Here's how the part is built. I have some questions about the finished solid (model axes, mm). Give positions to 0.01 mm unless a question says otherwise; leave off trailing zeros. Loops run counter-clockwise (first coordinate to the right, second up) from the corner with the lowest first, then second, coordinate; pieces in that order, holes last. Notation, with made-up numbers: (2, 73) -> (28, 73) arc R10 cw to (28, 79) -> close; hole circle Ø3 at (2.5, -16.75). An arc over 180 degrees is marked (long way). Answer in a Markdown table with one row per item. Add a question column.
Item 1: If we section it at B-B (z = -5): Write out the boundary of the cut face in (x, y) (3 decimals), then the cut area to 3 significant figures.
Item 2: If I drill on line 1 (Z direction, x = 25, y = -1.8); line 2 (Z direction, x = 23.75, y = -1.7), over which ranges is the centre line in solid material (lowest first)?
Item 3: If we section it at D-D (z = -16): Write out the boundary of the cut face in (x, y) (3 decimals).
Item 4: If we section it at C-C (y = -1.4): Give the number of separate pieces and of enclosed holes in the cut face, then the cut area to 3 significant figures.
Item 5: If we section it at A-A (x = 15): Write out the boundary of the cut face in (y, z) (3 decimals).
Item 6: For P1, Ø3.5, axis at x = 15, z = -15, coming from the -Y side (3 decimals); P2, Ø3, axis at x = 25, z = -35, coming from the +Y side, each with a flat end and sliding along its axis, tell me the tip position at first contact or that it passes through.
Item 7: We'd pull the mould along Z, two halves only. Please class faces 1 (the face through (13.4, -1.57, -24.93)), 2 (the face through (15, -3.175, -20)), 3 (the face through (15, -2, 0)): released by +Z, released by -Z, zero draft, split by the parting line, or undercut.
```python
from build123d import *

# Parameters (mm, degrees)
F0_R     = 1.6
F1_DEPTH = 3.175


# Not quite as in the source:
# - a length typed as a fraction of an inch, garbled in the dataset ("3 / 203.2 mm" for 3/8 in), is restored


with BuildPart() as f1:
    # F0 (on Front) → F1 (new body)
    with BuildSketch(Plane.XZ):
        with BuildLine():
            Line((27.46, 0), (2.54, 0))
            ThreePointArc((2.54, 0), (0.7439487758, -0.7439487758), (0, -2.54))
            Line((0, -2.54), (0, -37.46))
            ThreePointArc((0, -37.46), (0.7439487758, -39.2560512242), (2.54, -40))
            Line((2.54, -40), (27.46, -40))
            ThreePointArc((27.46, -40), (29.2560512242, -39.2560512242), (30, -37.46))
            Line((30, -37.46), (30, -2.54))
            ThreePointArc((30, -2.54), (29.2560512242, -0.7439487758), (27.46, 0))
        make_face()
        with Locations((5, -35)):
            Circle(F0_R, mode=Mode.SUBTRACT)
        with Locations((5, -25)):
            Circle(F0_R, mode=Mode.SUBTRACT)
        with Locations((15, -35)):
            Circle(F0_R, mode=Mode.SUBTRACT)
        with Locations((25, -35)):
            Circle(F0_R, mode=Mode.SUBTRACT)
        with Locations((15, -25)):
            Circle(F0_R, mode=Mode.SUBTRACT)
        with Locations((25, -25)):
            Circle(F0_R, mode=Mode.SUBTRACT)
        with Locations((5, -15)):
            Circle(F0_R, mode=Mode.SUBTRACT)
        with Locations((5, -5)):
            Circle(F0_R, mode=Mode.SUBTRACT)
        with Locations((15, -15)):
            Circle(F0_R, mode=Mode.SUBTRACT)
        with Locations((25, -15)):
            Circle(F0_R, mode=Mode.SUBTRACT)
        with Locations((15, -5)):
            Circle(F0_R, mode=Mode.SUBTRACT)
        with Locations((25, -5)):
            Circle(F0_R, mode=Mode.SUBTRACT)
    extrude(amount=F1_DEPTH)


solid = f1.part
```
Recorded:
| question | item | result |
|---|---|---|
| 1 | outline | (0, -3.175) -> (3.4, -3.175) -> (3.4, 0) -> (0, 0) -> close; (6.6, -3.175) -> (13.4, -3.175) -> (13.4, 0) -> (6.6, 0) -> close; (16.6, -3.175) -> (23.4, -3.175) -> (23.4, 0) -> (16.6, 0) -> close; (26.6, -3.175) -> (30, -3.175) -> (30, 0) -> (26.6, 0) -> close |
| 1 | area | 64.8 mm^2 |
| 2 | line 1 | z = -40 to -36.6, -33.4 to -26.6, -23.4 to -16.6, -13.4 to -6.6, -3.4 to 0 |
| 2 | line 2 | z = -40 to -36, -34 to -26, -24 to -16, -14 to -6, -4 to 0 |
| 3 | outline | (0, -3.175) -> (3.751, -3.175) -> (3.751, 0) -> (0, 0) -> close; (6.249, -3.175) -> (13.751, -3.175) -> (13.751, 0) -> (6.249, 0) -> close; (16.249, -3.175) -> (23.751, -3.175) -> (23.751, 0) -> (16.249, 0) -> close; (26.249, -3.175) -> (30, -3.175) -> (30, 0) -> (26.249, 0) -> close |
| 4 | separate pieces | 1 |
| 4 | enclosed holes | 12 |
| 4 | area | 1,100 mm^2 |
| 5 | outline | (-3.175, -40) -> (0, -40) -> (0, -36.6) -> (-3.175, -36.6) -> close; (-3.175, -33.4) -> (0, -33.4) -> (0, -26.6) -> (-3.175, -26.6) -> close; (-3.175, -23.4) -> (0, -23.4) -> (0, -16.6) -> (-3.175, -16.6) -> close; (-3.175, -13.4) -> (0, -13.4) -> (0, -6.6) -> (-3.175, -6.6) -> close; (-3.175, -3.4) -> (0, -3.4) -> (0, 0) -> (-3.175, 0) -> close |
| 6 | P1 | stops at y = -3.175 |
| 6 | P2 | passes through |
| 7 | face 1 | undercut |
| 7 | face 2 | zero draft |
| 7 | face 3 | released by +Z |
